from build123d import *

# Parameters (mm, degrees)
MODEL_W                 = 50.46
MODEL_H                 = 128.4
MODEL_R                 = 1.25
MODEL_R_2               = 1.45
BOSS_EXTRU_1_DEPTH      = 2.5
CHANFREIN1_SIZE         = 1.4
ESQUISSE1_R             = 1.4
ESQUISSE1_R_2           = 2
ENL_V_MAT_EXTRU_1_DEPTH = 138.98196114


with BuildPart() as part:
    # Model → Boss.-Extru.1 (new body)
    with BuildSketch(Plane.XY):
        with Locations((25.23, 64.2)):
            Rectangle(MODEL_W, MODEL_H)
        with Locations((2.37, 14.7)):
            Circle(MODEL_R, mode=Mode.SUBTRACT)
        with Locations((12.53, 14.7)):
            Circle(MODEL_R, mode=Mode.SUBTRACT)
        with Locations(Location((37.93, 14.7, 0), (0, 0, 180))):
            Circle(MODEL_R, mode=Mode.SUBTRACT)
        with Locations((7.45, 14.7)):
            Circle(MODEL_R, mode=Mode.SUBTRACT)
        with Locations((7.45, 113.7)):
            Circle(MODEL_R_2, mode=Mode.SUBTRACT)
        with Locations((17.61, 14.7)):
            Circle(MODEL_R, mode=Mode.SUBTRACT)
        with Locations(Location((43.01, 14.7, 0), (0, 0, 180))):
            Circle(MODEL_R, mode=Mode.SUBTRACT)
        with Locations(Location((48.09, 14.7, 0), (0, 0, 180))):
            Circle(MODEL_R, mode=Mode.SUBTRACT)
        with BuildLine():
            Line((9.895403852, 123.75), (5.004596148, 123.75))
            ThreePointArc((5.004596148, 123.75), (4.5, 125.4), (5.004596148, 127.05))
            Line((5.004596148, 127.05), (9.895403852, 127.05))
            ThreePointArc((9.895403852, 127.05), (10.4, 125.4), (9.895403852, 123.75))
        make_face(mode=Mode.SUBTRACT)
        with BuildLine():
            Line((9.895403852, 1.35), (5.004596148, 1.35))
            ThreePointArc((5.004596148, 1.35), (4.5, 3), (5.004596148, 4.65))
            Line((5.004596148, 4.65), (9.895403852, 4.65))
            ThreePointArc((9.895403852, 4.65), (10.4, 3), (9.895403852, 1.35))
        make_face(mode=Mode.SUBTRACT)
        with BuildLine():
            Line((40.564596148, 1.35), (45.455403852, 1.35))
            ThreePointArc((45.455403852, 1.35), (45.96, 3), (45.455403852, 4.65))
            Line((45.455403852, 4.65), (40.564596148, 4.65))
            ThreePointArc((40.564596148, 4.65), (40.06, 3), (40.564596148, 1.35))
        make_face(mode=Mode.SUBTRACT)
        with BuildLine():
            Line((40.564596148, 123.75), (45.455403852, 123.75))
            ThreePointArc((45.455403852, 123.75), (45.96, 125.4), (45.455403852, 127.05))
            Line((45.455403852, 127.05), (40.564596148, 127.05))
            ThreePointArc((40.564596148, 127.05), (40.06, 125.4), (40.564596148, 123.75))
        make_face(mode=Mode.SUBTRACT)
    extrude(amount=BOSS_EXTRU_1_DEPTH)

    # Chanfrein1
    chanfrein1_edges = [part.edges().sort_by_distance(p)[0] for p in [
        (6, 113.7, 2.5),
    ]]
    chamfer(chanfrein1_edges, length=CHANFREIN1_SIZE)

    # Esquisse1 → Enlèv. mat.-Extru.1 (cut, through all)
    with BuildSketch(Plane.XY.offset(2.5)):
        with Locations((18.887367925, 27.211559267)):
            Circle(ESQUISSE1_R)
        with Locations((7.900573508, 27.200461502)):
            Circle(ESQUISSE1_R_2)
    extrude(amount=-ENL_V_MAT_EXTRU_1_DEPTH, mode=Mode.SUBTRACT)


solid = part.part
Design review of the part built by this model. Coordinates are the model's own, in mm. A direction names the side the tool comes from. Round coordinates to 2 decimals unless told otherwise and drop trailing zeros. Write each loop counter-clockwise with the first axis right and the second up, starting at its lowest first coordinate (ties: lowest second). Pieces come first, ordered by that corner, then holes. Notation, with made-up numbers: (80.5, -10.75) -> (118.5, -10.75) arc R18 ccw to (118.5, -3.75) -> close; hole circle Ø1 at (61.25, 34). An arc over 180 degrees is marked (long way). One line per item, written item: value. Start each with the question number.
Q1. Add section C-C (x = 12.53). Give the boundary of the cut face in (y, z).
Q2. Tool access review of faces 4 (the face through (4.5, 125.4, 1.2)), 5 (the face through (25, 65, 2.5)): name each direction out of +Z, -Z, +X, -X, +Y, -Y from which nothing blocks a thin tool from reaching the whole face with its end or side.
Q3. Insertion check: P1, Ø2, axis at x = 17.61, y = 14.7, coming from the +Z side. The pin has a flat end and moves straight along its axis. Give the tip position at first contact, or say it passes through.
Q4. The part is to be moulded in two halves that separate along X. For faces 1 (the face through (50.46, 63, 1)), 2 (the face through (0, 63, 1)), 3 (the face through (43, 127.05, 1)), say which applies: pulls with the +X half, pulls with the -X half, needs draft (parallel to the pull), parting line crosses it, or undercut.
Q5. Add section B-B (x = 43.01). Give the boundary of the cut face in (y, z).
Q6. Add section A-A (y = 113.7). Give the boundary of the cut face in (x, z).
Q7. Add section D-D (z = 0.5). State how many separate pieces and enclosed holes the cut face has, then the cut area to 3 significant figures.
Q8. To check wall thickness, follow probe 1 along Y at (x, z) = (45, 1.75); probe 2 along Y at (x, z) = (43.01, 0.85); probe 3 along Y at (x, z) = (17.61, 1.65). State the ranges of each line that lie inside material, in increasing order.
Response:
1. outline: (0, 0) -> (13.45, 0) -> (13.45, 2.5) -> (0, 2.5) -> close; (15.95, 0) -> (128.4, 0) -> (128.4, 2.5) -> (15.95, 2.5) -> close
2. face 4: +Z, -Z
2. face 5: +Z, +X, -X, +Y, -Y
3. P1: passes through
4. face 1: pulls with the +X half
4. face 2: pulls with the -X half
4. face 3: undercut
5. outline: (0, 0) -> (1.35, 0) -> (1.35, 2.5) -> (0, 2.5) -> close; (4.65, 0) -> (13.45, 0) -> (13.45, 2.5) -> (4.65, 2.5) -> close; (15.95, 0) -> (123.75, 0) -> (123.75, 2.5) -> (15.95, 2.5) -> close; (127.05, 0) -> (128.4, 0) -> (128.4, 2.5) -> (127.05, 2.5) -> close
6. outline: (0, 0) -> (6, 0) -> (6, 1.1) -> (4.6, 2.5) -> (0, 2.5) -> close; (8.9, 0) -> (50.46, 0) -> (50.46, 2.5) -> (10.3, 2.5) -> (8.9, 1.1) -> close
7. separate pieces: 1
7. enclosed holes: 14
7. area: 6,350 mm^2
8. probe 1: y = 0 to 1.35, 4.65 to 123.75, 127.05 to 128.4
8. probe 2: y = 0 to 1.35, 4.65 to 13.45, 15.95 to 123.75, 127.05 to 128.4
8. probe 3: y = 0 to 13.45, 15.95 to 26.64, 27.78 to 128.4
